Can you work these out from the model? Positions are in its coordinate system, mm. A direction names the side the tool comes from. Give positions to 0.01 mm unless a question says otherwise; leave off trailing zeros. Order: outer loops, then holes, each group sorted by start corner. A loop starts at its lowest first (then second) coordinate and runs counter-clockwise, first axis right, second up. Notation, with made-up numbers: M 42,-25 L 86,-25 A24 ccw 86,10 Z; hole C 74.25,-21.75 d5. An arc over 180 degrees is marked long. Answer as a JSON object with one key per item and string values.
```python
from build123d import *

# Parameters (mm, degrees)
SKETCH1_W            = 40.40124
SKETCH1_H            = 34.036
SKETCH1_R            = 1.257288094
BOSS_EXTRUDE1_DEPTH  = 4.7625
M6_CLEARANCE_HOLE1_D = 7
BOSS_EXTRUDE3_DEPTH  = 6.35


with BuildPart() as part:
    # Sketch1 → Boss-Extrude1 (new body)
    with BuildSketch(Plane(origin=(0, 0, 0), x_dir=(1, 0, 0), z_dir=(0, 1, 0))):
        with Locations((20.20062, 17.018)):
            Rectangle(SKETCH1_W, SKETCH1_H)
        with Locations(Location((20.20062, 25.522416525, 0), (0, 0, 90))):
            Circle(SKETCH1_R, mode=Mode.SUBTRACT)
    extrude(amount=BOSS_EXTRUDE1_DEPTH)

    # M6 Clearance Hole1 (through all)
    with Locations(Plane(origin=(0, 4.7625, 0), x_dir=(1, 0, 0), z_dir=(0, 1, 0))):
        with Locations((20.20062, 25.522416525)):
            Hole(M6_CLEARANCE_HOLE1_D / 2)

    # Sketch5 → Boss-Extrude3 (add)
    with BuildSketch(Plane(origin=(40.40124, 0, 0), x_dir=(0, 0, -1), z_dir=(1, 0, 0))):
        with BuildLine():
            Line((0, 4.7625), (34.036, 4.7625))
            ThreePointArc((34.036, 4.7625), (12.064122693, 17.098372866), (-13.078907049, 15.43548166))
            ThreePointArc((-13.078907049, 15.43548166), (-4.343178895, 12.790354185), (0, 4.7625))
        make_face()
    boss_extrude3 = extrude(amount=-BOSS_EXTRUDE3_DEPTH)

    # Mirror1: Boss-Extrude3 across plane
    add(boss_extrude3.mirror(Plane(origin=(20.20062, 0, 0), x_dir=(0, 0, 1), z_dir=(1, 0, 0))))


solid = part.part
```
1) I want a section at B-B on y = 9.5. Write out the boundary of the cut face in (x, z).
Results found:
{"outline": "M 0,-28.62 L 6.35,-28.62 L 6.35,1.54 L 0,1.54 Z; M 34.05,-28.62 L 40.4,-28.62 L 40.4,1.54 L 34.05,1.54 Z"}
2) I need wall thicknesses on L1, parallel to X at y = 11.25, z = -18.5; L2, parallel to Z at x = 2, y = 4.25; L3, parallel to Y at x = 26, z = -4. Which ranges of each line are inside material? Lowest first, please.
Results found:
{"L1": "x = 0 to 6.35, 34.05 to 40.4", "L2": "z = -34.04 to 0", "L3": "y = 0 to 4.76"}
3) I'm going to push flat-ended pins straight in: pin 1 Ø2.5 at (x, y) = (19.5, 3.5) entering from +Z; pin 2 Ø8 at (x, y) = (9.5, 4.5) entering from +Z (3 decimals); pin 3 Ø14 at (x, z) = (15, -20.5) entering from +Y. Where does each tip first touch, or does it pass through?
Results found:
{"pin 1": "stops at z = 0", "pin 2": "stops at z = 0.445", "pin 3": "stops at y = 4.76"}
4) Thinking about a two-plate mould opening in Z: for faces 4 (the face through (16.86, 2.35, -26.57)), 5 (the face through (20, 4.762, -17)), 6 (the face through (37.27, 17.02, -12.41)), 7 (the face through (20, 2, -34.036)), which applies, pulls with the +Z half, pulls with the -Z half, needs draft (parallel to the pull), parting line crosses it, or undercut?
Results found:
{"face 4": "undercut", "face 5": "needs draft", "face 6": "parting line crosses it", "face 7": "pulls with the -Z half"}
5) I want a section at D-D on z = -7.5. Write out the boundary of the cut face in (x, y).
Results found:
{"outline": "M 0,0 L 40.4,0 L 40.4,17.88 L 34.05,17.88 L 34.05,4.76 L 6.35,4.76 L 6.35,17.88 L 0,17.88 Z"}
6) I want a section at A-A on z = 9. Write out the boundary of the cut face in (x, y).
Results found:
{"outline": "M 0,15.13 L 6.35,15.13 L 6.35,16.73 L 0,16.73 Z; M 34.05,15.13 L 40.4,15.13 L 40.4,16.73 L 34.05,16.73 Z"}
7) I want a section at C-C on x = 15.5. Write out the boundary of the cut face in (y, z), and give its area (3 significant figures).
Results found:
{"outline": "M 0,-34.04 L 4.76,-34.04 L 4.76,0 L 0,0 Z", "area": "162 mm²"}
8) For faces 1 (the face through (34.051, 12, -10)), 2 (the face through (3.13, 17.02, -12.41)), 3 (the face through (20, 2, 0)), which set-ups out of +Z, -Z, +X, -X, +Y, -Y let a thin tool reach every point of the face, with its end or its side?
Results found:
{"face 1": "+Z, -Z, +Y", "face 2": "+X, -X, +Y", "face 3": "+Z, +X, -X, -Y"}
